Could you check a few things on this model? Use its own coordinates, in mm. Face numbers are marked on the shaded views. A direction names the side the tool comes from. Coordinates: 2 decimals unless noted, no trailing zeros. Order: outer loops, then holes, each group sorted by start corner. A loop starts at its lowest first (then second) coordinate and runs counter-clockwise, first axis right, second up. Notation, with made-up numbers: (76.25, -10.5) -> (81.25, -10.5) arc R18 cw to (81.25, 20.5) -> close; hole circle Ø5 at (2, 89.25). An arc over 180 degrees is marked (long way). Use a Markdown table: item, result. Add a question column.
1) Which directions (+Z, -Z, +X, -X, +Y, -Y) give clear straight access to the entire face, cutting with the end or side of a thin tool? Please do the marked faces 1 and 2.
2) If we section it at B-B (z = -87): Write out the boundary of the cut face in (x, y), plus the area to 3 significant figures.
3) Will these pins go through, and if not, where does the flat tip stop? pin 1 Ø2 at (x, z) = (-7, -74) entering from -Y; pin 2 Ø1.5 at (y, z) = (-3.5, -51) entering from -X; pin 3 Ø1 at (y, z) = (3, -48.5) entering from +X; pin 4 Ø8 at (y, z) = (-1, -47.5) entering from -X.
4) If I drill on L1, parallel to Z at x = -5.25, y = 0.75; L2, parallel to Y at x = 0, z = -80; L3, parallel to Y at x = -3.25, z = -42.5, over which ranges is the centre line in solid material (lowest first)? Write a range as [from, to].
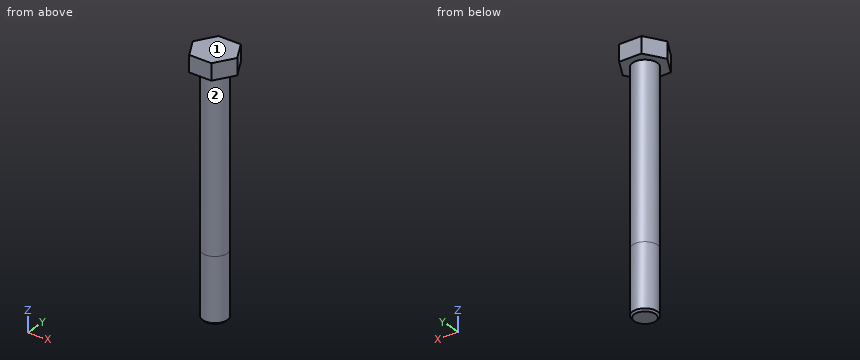
Solid Edge part; units mm, degrees
sketch "Sketch1" plane through (0, 0, 0) normal (0, 0, 1) x (1, 0, 0)
  circle A0 centre (0, 0) radius 9.28
extrude "Protrusion1" add sketch "Sketch1" along normal blind 6.63
sketch "Sketch2" plane through (0, 0, 0) normal (0, 0, -1) x (1, 0, 0)
  circle A0 centre (0, 0) radius 5
extrude "Protrusion2" add sketch "Sketch2" along normal blind 95
sketch "Sketch3" plane through (0, 0, -95) normal (0, 0, -1) x (1, 0, 0)
  circle A0 centre (0, 0) radius 4.9997
extrude "Cutout1" cut sketch "Sketch3" against normal blind 26 flip side to cut
chamfer "Chamfer_1" distance 0.75 angle 45 1 edges at (-4.9997, 0, -95)
sketch "Sketch4" plane through (0, 0, 6.63) normal (0, 0, 1) x (1, 0, 0)
  line L0 (-4.703, 8) -> (4.703, 8)
extrude "Cutout2" cut sketch "Sketch4" against normal up to next material side at (0, 8.05, 6.63)
pattern_circular "Pattern1" count 6 over 360 about axis through (0, 0, 6.63) along (0, 0, 1) of "Cutout2"
properties part number "185550" material "Stainless Steel, 304"
Answer sheet:
| question | item | result |
|---|---|---|
| 1 | face 1 | +Z, +X, -X, +Y, -Y |
| 1 | face 2 | -Z |
| 2 | outline | circle Ø10 at (0, 0) |
| 2 | area | 78.5 mm2 |
| 3 | pin 1 | through |
| 3 | pin 2 | x = -4.18 |
| 3 | pin 3 | x = 4.33 |
| 3 | pin 4 | x = -5 |
| 4 | L1 | [0, 6.63] |
| 4 | L2 | [-5, 5] |
| 4 | L3 | [-3.8, 3.8] |
